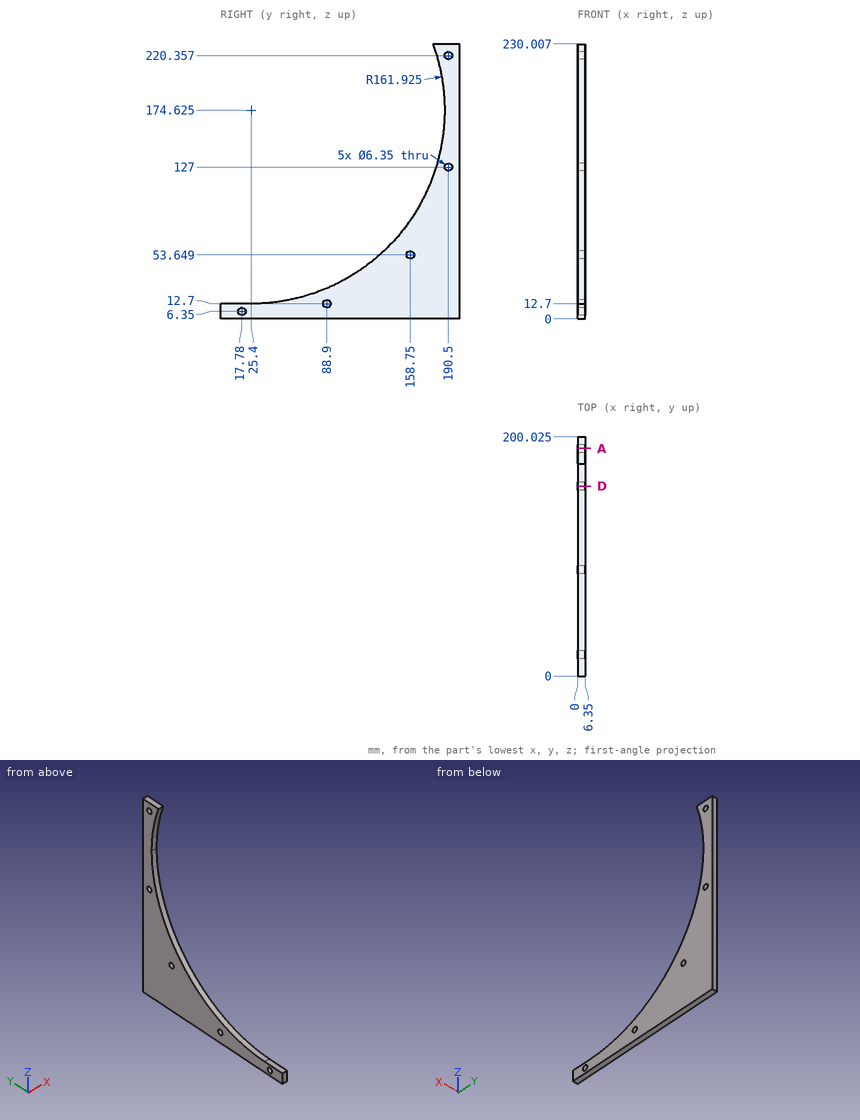
Design review of the part shown in the three views and the two pictorial views. Dimensions are in mm from the part's minimum x, y and z. Coordinates: 2 decimals unless noted, no trailing zeros. Order: outer loops, then holes, each group sorted by start corner. A loop starts at its lowest first (then second) coordinate and runs counter-clockwise, first axis right, second up.
1) Clearance check with flat-ended pins moving along their axes: pin 1 (1 mm diameter, centred on x = 2.5, z = 43.5, fed in from -Y); pin 2 (3 mm diameter, centred on x = 3.5, y = 16, fed in from +Z); pin 3 (3 mm diameter, centred on x = 1, z = 69, fed in from -Y) (1 decimal). State where each tip first meets the part, or that it passes through.
2) Wall thickness on line 1 along Z through (x, y) = (3, 190.5) (1 decimal); line 2 along Y through (x, z) = (2.25, 87.5) (1 decimal); line 3 along Y through (x, z) = (5, 12) (1 decimal): over which ranges is each line inside the solid? List them lowest first.
3) Take a section at A-A, the plane y = 190.5. State how many separate pieces and enclosed holes the cut face has, and give its area (3 significant figures).
4) Take a section at D-D, the plane y = 158.75. Give the boundary of the cut face in (x, z).
Returned:
1. pin 1: stops at y = 119.71
1. pin 2: stops at z = 12.7
1. pin 3: stops at y = 146.8
2. line 1: z = 0 to 123.8, 130.2 to 217.2, 223.5 to 230
2. line 2: y = 161.9 to 200
2. line 3: y = 0 to 85.8, 92 to 200
3. separate pieces: 3
3. enclosed holes: 0
3. area: 1,380 mm2
4. outline: (0, 0) - (6.35, 0) - (6.35, 50.47) - (0, 50.47) - close; (0, 56.82) - (6.35, 56.82) - (6.35, 82.77) - (0, 82.77) - close
